The model under review builds one solid part; all positions refer to its coordinate system, in mm. Face numbers are marked on the shaded views. A direction names the side the tool comes from. Give positions to 0.01 mm unless a question says otherwise; leave off trailing zeros. Order: outer loops, then holes, each group sorted by start corner. A loop starts at its lowest first (then second) coordinate and runs counter-clockwise, first axis right, second up. Notation, with made-up numbers: (-24, 5) - (-3, 5) arc R25 cw to (-3, 37) - close; hole circle Ø1 at (46.5, 84). An arc over 180 degrees is marked (long way). Use CSV: the item, a comma, the result in double quotes. Start each with the question number.
1. Take a section at C-C, the plane x = 40.5. State the section outline as (y, z) points, then the cut area to 3 significant figures.
2. Machinability: for the marked faces 1 and 2, which of the approach directions +Z, -Z, +X, -X, +Y, -Y give a long, thin tool a straight path to every point of the face, cutting with its end or side? Answer none if there is none.
3. Take a section at A-A, the plane z = 0. State the section outline as (x, y) points, then the cut area to 4 significant figures.
4. Take a section at B-B, the plane x = 0. State the section outline as (y, z) points.
5. Take a section at D-D, the plane z = -40. State the section outline as (x, y) points.
6. For pin 1 (7.5 mm diameter, centred on x = -2, y = -4, fed in from +Z); pin 2 (16.5 mm diameter, centred on y = -11, z = -12.5, fed in from -X), all flat-tipped, find the tip position at first contact; note any pin that passes through.
7. Draft analysis for pull direction Z (two halves, no side actions). For the marked faces 3, 4, 5 and 6, state which applies: released by +Z, released by -Z, zero draft, split by the parting line, or undercut.
8. To check wall thickness, follow line 1 (Z direction, x = -27, y = 63.5); line 2 (Y direction, x = 50, z = 10.5). State the ranges of each line that lie inside material, in increasing order. Write a range as [from, to].
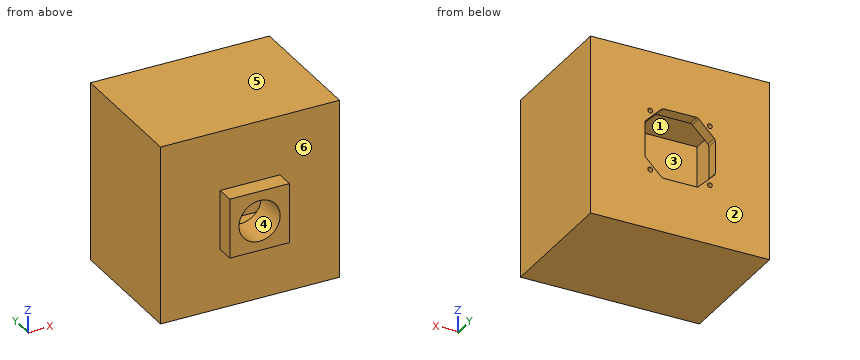
```python
from build123d import *

# Parameters (mm, degrees)
F0_W      = 150
F0_H      = 150
F1_DEPTH  = 100
F2_W      = 130
F2_H      = 130
F3_DEPTH  = 85
F4_W      = 150
F4_H      = 150
F5_DEPTH  = 10
F6_W      = 50
F6_H      = 50
F7_DEPTH  = 15
F8_R      = 17.25
F9_DEPTH  = 30
F10_R     = 2
F11_DEPTH = 10
F13_DEPTH = 10
F14_R     = 3


with BuildPart() as f1:
    # F0 (on Front) → F1 (new body)
    with BuildSketch(Plane.XZ):
        Rectangle(F0_W, F0_H)
    extrude(amount=-F1_DEPTH)

    # F2 (on face) → F3 (cut)
    with BuildSketch(Plane(origin=(0, 100, 0), x_dir=(-1, 0, 0), z_dir=(0, 1, 0))):
        Rectangle(F2_W, F2_H)
    extrude(amount=-F3_DEPTH, mode=Mode.SUBTRACT)

    # F4 (on face) → F5 (join)
    with BuildSketch(Plane(origin=(0, 100, 0), x_dir=(-1, 0, 0), z_dir=(0, 1, 0))):
        Rectangle(F4_W, F4_H)
    extrude(amount=F5_DEPTH)

    # F6 (on face) → F7 (join)
    with BuildSketch(Plane.XZ):
        Rectangle(F6_W, F6_H)
    extrude(amount=F7_DEPTH)

    # F8 (on face) → F9 (cut, through all)
    with BuildSketch(Plane.XZ.offset(15)):
        Circle(F8_R)
    extrude(amount=-F9_DEPTH, mode=Mode.SUBTRACT)

    # F10 (on face) → F11 (cut, through all)
    with BuildSketch(Plane(origin=(0, 110, 0), x_dir=(-1, 0, 0), z_dir=(0, 1, 0))):
        with Locations((25, 25)):
            Circle(F10_R)
        with Locations((25, -25)):
            Circle(F10_R)
        with Locations((-25, 25)):
            Circle(F10_R)
        with Locations((-25, -25)):
            Circle(F10_R)
    extrude(amount=-F11_DEPTH, mode=Mode.SUBTRACT)

    # F12 (on face) → F13 (cut, through all)
    with BuildSketch(Plane(origin=(0, 110, 0), x_dir=(-1, 0, 0), z_dir=(0, 1, 0))):
        Polygon((14.85, 29.471261), (-14.85, 29.471261), (-29.5, 14.85), (-29.5, -14.85), (-14.85, -29.471261), (14.85, -29.471261), (29.5, -14.85), (29.5, 14.85), align=None)
    extrude(amount=-F13_DEPTH, mode=Mode.SUBTRACT)

    # F14
    f14_edges = [f1.edges().sort_by_distance(p)[0] for p in [
        (29.5, 105, 14.85),
        (14.85, 105, 29.471261),
        (29.5, 105, -14.85),
        (14.85, 105, -29.471261),
        (-14.85, 105, -29.471261),
        (-14.85, 105, 29.471261),
        (-29.5, 105, 14.85),
        (-29.5, 105, -14.85),
    ]]
    fillet(f14_edges, radius=F14_R)


solid = f1.part
```
Determined:
1,outline,"(0, -75) - (110, -75) - (110, 75) - (0, 75) - close; hole (15, -65) - (100, -65) - (100, 65) - (15, 65) - close"
1,area,"5,450 mm²"
2,face 1,"none"
2,face 2,"+Z, -Z, +X, -X, +Y"
3,outline,"(-75, 0) - (-25, 0) - (-25, -15) - (-17.25, -15) - (-17.25, 15) - (-65, 15) - (-65, 100) - (-29.5, 100) - (-29.5, 110) - (-75, 110) - close; (17.25, -15) - (25, -15) - (25, 0) - (75, 0) - (75, 110) - (29.5, 110) - (29.5, 100) - (65, 100) - (65, 15) - (17.25, 15) - close"
3,area,"4,575 mm²"
4,outline,"(-15, -25) - (0, -25) - (0, -75) - (110, -75) - (110, -29.47) - (100, -29.47) - (100, -65) - (15, -65) - (15, -17.25) - (-15, -17.25) - close; (-15, 17.25) - (15, 17.25) - (15, 65) - (100, 65) - (100, 29.47) - (110, 29.47) - (110, 75) - (0, 75) - (0, 25) - (-15, 25) - close"
5,outline,"(-75, 0) - (75, 0) - (75, 110) - (-75, 110) - close; hole (-65, 15) - (65, 15) - (65, 100) - (-65, 100) - close"
6,pin 1,"stops at z = 25"
6,pin 2,"stops at x = -25"
7,face 3,"undercut"
7,face 4,"undercut"
7,face 5,"released by +Z"
7,face 6,"zero draft"
8,line 1,"z = [-75, -65], [65, 75]"
8,line 2,"y = [0, 15], [100, 110]"
